Input: part model. Units: mm. Frame: model coordinates. Coordinates: 2 decimals unless noted, no trailing zeros. Loops run counter-clockwise (first coordinate to the right, second up) from the corner with the lowest first, then second, coordinate; pieces in that order, holes last.
(1) Section D-D, the plane z = 688.5. Return loops of the section in (x, y).
(2) Contact query for a flat-ended pin moving along its axis: P1, Ø5.5, axis at x = 11.5, z = 371, coming from the +Y side. Output: stop coordinate, or through.
(3) Section C-C, the plane y = 55. Return loops of the section in (x, z).
(4) Line query: L1, parallel to Z at x = 6, y = 250; L2, parallel to Z at x = 16, y = 250; L3, parallel to Z at x = 12.25, y = 164. Output: solid intervals per line, ascending.
(5) Section B-B, the plane x = 13. Return loops of the section in (y, z), then the cut area to 3 significant figures.
(6) Section A-A, the plane z = 205. Return loops of the section in (x, y), then the cut area to 3 significant figures.
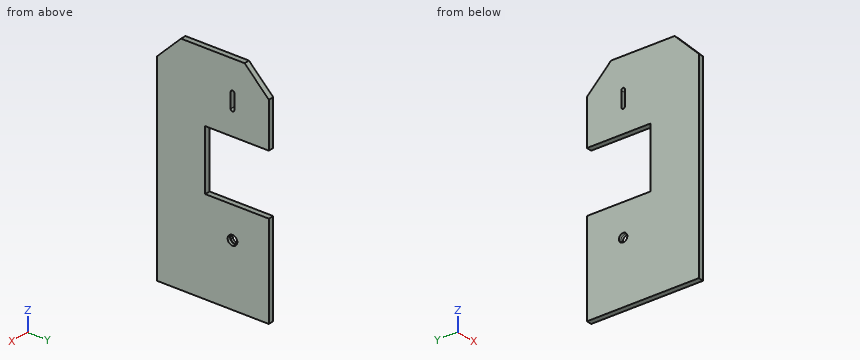
```python
from build123d import *

# Parameters (mm, degrees)
F0_R     = 6
F1_DEPTH = 18
F2_SIZE  = 80
F3_R     = 16
F4_DEPTH = 10
F5_R     = 14
F6_DEPTH = 8


with BuildPart() as f1:
    # F0 (on Right) → F1 (new body)
    with BuildSketch(Plane.YZ):
        Polygon((0, 740), (0, 0), (370, 0), (370, 310), (160, 310), (160, 510), (370, 510), (370, 740), align=None)
        with Locations((250, 205)):
            Circle(F0_R, mode=Mode.SUBTRACT)
        with BuildLine():
            ThreePointArc((244.026492, 640.563206), (250.281914, 645.993373), (256, 640))
            Line((256, 640), (256, 590))
            ThreePointArc((256, 590), (250.281914, 584.006627), (244.026492, 589.436794))
            ThreePointArc((244.026492, 589.436794), (244, 590), (244.026492, 590.563206))
            Line((244.026492, 590.563206), (244.026492, 639.436794))
            ThreePointArc((244.026492, 639.436794), (244, 640), (244.026492, 640.563206))
        make_face(mode=Mode.SUBTRACT)
    extrude(amount=F1_DEPTH)

    # F2
    f2_edges = [f1.edges().sort_by_distance(p)[0] for p in [
        (9, 0, 740),
        (9, 370, 740),
    ]]
    chamfer(f2_edges, length=F2_SIZE)

    # F3 (on face) → F4 (cut)
    with BuildSketch(Plane.YZ.offset(18)):
        with Locations((250, 205)):
            Circle(F3_R)
    extrude(amount=-F4_DEPTH, mode=Mode.SUBTRACT)

    # F5 (on face) → F6 (cut)
    with BuildSketch(Plane(origin=(0, 0, 0), x_dir=(0, -1, 0), z_dir=(-1, 0, 0))):
        with Locations((-250, 205)):
            Circle(F5_R)
    extrude(amount=-F6_DEPTH, mode=Mode.SUBTRACT)


solid = f1.part
```
Report:
1. outline: (0, 28.5) - (18, 28.5) - (18, 341.5) - (0, 341.5) - close
2. P1: stops at y = 160
3. outline: (0, 0) - (18, 0) - (18, 715) - (0, 715) - close
4. L1: z = 0 to 191, 219 to 310, 510 to 584, 646 to 740
4. L2: z = 0 to 189, 221 to 310, 510 to 584, 646 to 740
4. L3: z = 0 to 310, 510 to 740
5. outline: (0, 0) - (370, 0) - (370, 310) - (160, 310) - (160, 510) - (370, 510) - (370, 660) - (290, 740) - (80, 740) - (0, 660) - close; hole circle Ø32 at (250, 205); hole (244.03, 589.44) arc R6 ccw to (256, 590) - (256, 640) arc R6 ccw to (244.03, 640.56) arc R6 ccw to (244.03, 639.44) - (244.03, 590.56) arc R6 ccw to start
5. area: 224,000 mm2
6. outline: (0, 0) - (18, 0) - (18, 234) - (8, 234) - (8, 236) - (0, 236) - close; (0, 264) - (8, 264) - (8, 266) - (18, 266) - (18, 370) - (0, 370) - close
6. area: 6,120 mm2
